Answer from the drawing. Dimensions are ordinates in mm from the lowest x, y and z of the part. A direction names the side the tool comes from. Round coordinates to 2 decimals unless told otherwise and drop trailing zeros. Write each loop counter-clockwise with the first axis right and the second up, starting at its lowest first coordinate (ties: lowest second). Pieces come first, ordered by that corner, then holes. Notation, with made-up numbers: (80, 8.5) - (102, 8.5) arc R23 ccw to (102, 27.5) - close; hole circle Ø6 at (13.25, -35). An arc over 180 degrees is marked (long way). Answer as CSV lines item,"result". Start each with the question number.
1) Consider line 1 along Z through (x, y) = (30.4, 9); line 2 along X through (y, z) = (7.25, 7.5); line 3 along X through (y, z) = (11, 17.9). Determine where each line is inside the solid, lowest interval first.
2) Find section A-A on y = 12. Determine the outline of the cut face in (x, z), then the cut area to 3 significant figures.
3) For a pull along Z with two mould halves and no side action, classify the marked faces 3, 4 and 5 as +Z half, -Z half, draft (parallel to the pull), parting line (faces both ways), or undercut.
4) Find section D-D on z = 3.5. Determine the outline of the cut face in (x, y), then the cut area to 3 significant figures.
5) Which of the six approach directions +Z, -Z, +X, -X, +Y, -Y give full straight-line access (tool end or side, diameter ignored) to the marked faces 1 and 2?
6) Find section B-B on z = 7.5. Determine the outline of the cut face in (x, y).
7) Each of these flat-tipped pins is pushed along its axis until it touches: pin 1 (5.5 mm diameter, centred on x = 5, z = 17.9, fed in from -Y); pin 2 (2 mm diameter, centred on x = 30.4, z = 7.5, fed in from -Y). Where does it stop, or does it pass through?
8) Find section C-C on y = 1.5. Determine the outline of the cut face in (x, z).
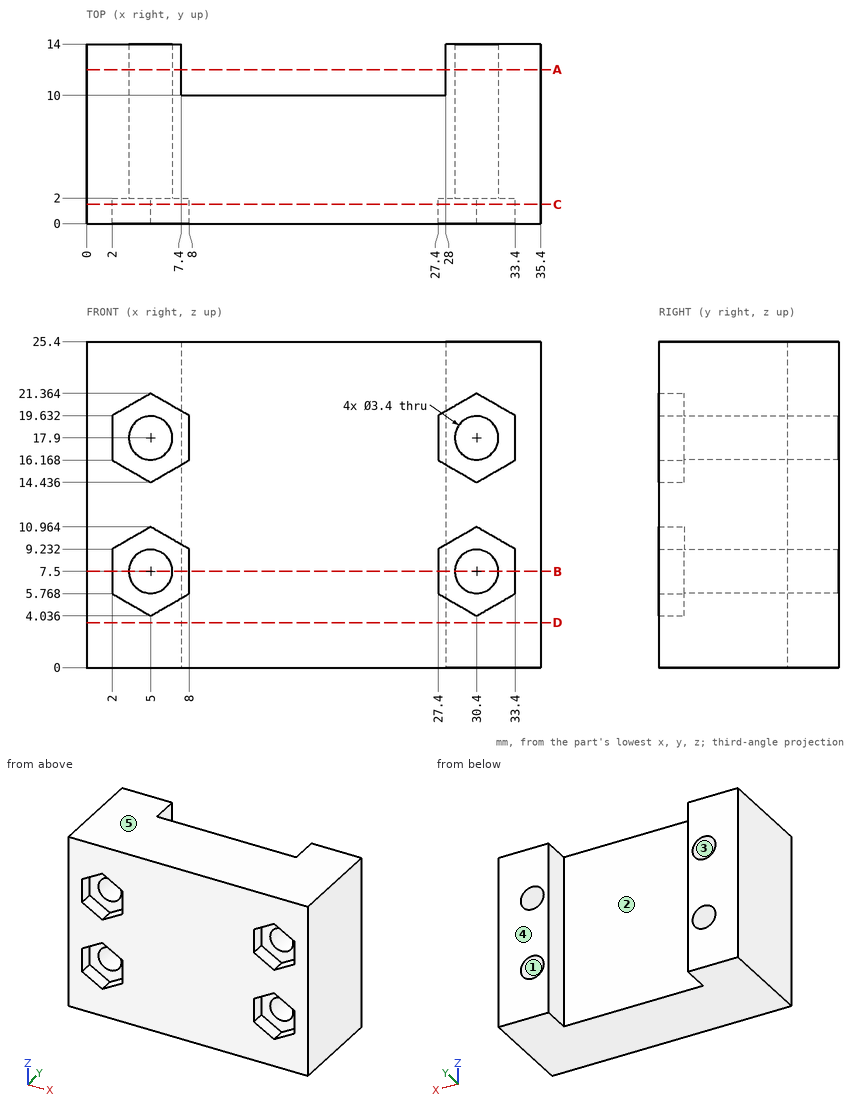
Check values:
1,line 1,"z = 0 to 5.8, 9.2 to 16.2, 19.6 to 25.4"
1,line 2,"x = 0 to 3.3, 6.7 to 28.7, 32.1 to 35.4"
1,line 3,"x = 0 to 3.3, 6.7 to 7.4, 28 to 28.7, 32.1 to 35.4"
2,outline,"(0, 0) - (7.4, 0) - (7.4, 25.4) - (0, 25.4) - close; (28, 0) - (35.4, 0) - (35.4, 25.4) - (28, 25.4) - close; hole circle Ø3.4 at (5, 7.5); hole circle Ø3.4 at (5, 17.9); hole circle Ø3.4 at (30.4, 7.5); hole circle Ø3.4 at (30.4, 17.9)"
2,area,"340 mm^2"
3,face 3,"undercut"
3,face 4,"draft"
3,face 5,"+Z half"
4,outline,"(0, 0) - (35.4, 0) - (35.4, 14) - (28, 14) - (28, 10) - (7.4, 10) - (7.4, 14) - (0, 14) - close"
4,area,"413 mm^2"
5,face 1,"+Y, -Y"
5,face 2,"+Z, -Z, +Y"
6,outline,"(0, 0) - (2, 0) - (2, 2) - (3.3, 2) - (3.3, 14) - (0, 14) - close; (6.7, 2) - (8, 2) - (8, 0) - (27.4, 0) - (27.4, 2) - (28.7, 2) - (28.7, 14) - (28, 14) - (28, 10) - (7.4, 10) - (7.4, 14) - (6.7, 14) - close; (32.1, 2) - (33.4, 2) - (33.4, 0) - (35.4, 0) - (35.4, 14) - (32.1, 14) - close"
7,pin 1,"stops at y = 2"
7,pin 2,"passes through"
8,outline,"(0, 0) - (35.4, 0) - (35.4, 25.4) - (0, 25.4) - close; hole (2, 5.77) - (5, 4.04) - (8, 5.77) - (8, 9.23) - (5, 10.96) - (2, 9.23) - close; hole (2, 16.17) - (5, 14.44) - (8, 16.17) - (8, 19.63) - (5, 21.36) - (2, 19.63) - close; hole (27.4, 5.77) - (30.4, 4.04) - (33.4, 5.77) - (33.4, 9.23) - (30.4, 10.96) - (27.4, 9.23) - close; hole (27.4, 16.17) - (30.4, 14.44) - (33.4, 16.17) - (33.4, 19.63) - (30.4, 21.36) - (27.4, 19.63) - close"
